from build123d import *

# Parameters (mm, degrees)
SKETCH1_W                  = 38.1
SKETCH1_H                  = 38.1
PRONG_HOLDERS_DEPTH        = 19.05
SKETCH5_R                  = 2.54
SCREW_HOLDER_DEPTH         = 58.15
GROOVE_CUT_OUT_DEPTH       = 58.15
SKETCH6_W                  = 38.1
SKETCH6_H                  = 31.75
OPENING_OF_THE_TOP_DEPTH   = 66.991135768
ROUNDING_OFF_HODER_EDGES_R = 19.05
SKETCH7_W                  = 38.1
SKETCH7_H                  = 38.1
ADJUSTABLE_LENGTH_DEPTH    = 25.4
SKETCH8_W                  = 5.08
SKETCH8_H                  = 38.1
BOSS_EXTRUDE3_DEPTH        = 25.4
SKETCH9_R                  = 2.54
CUT_EXTRUDE4_DEPTH         = 99.578509321


with BuildPart() as part:
    # Sketch1 → Prong holders (new, symmetric)
    with BuildSketch(Plane(origin=(0, 0, 0), x_dir=(1, 0, 0), z_dir=(0, 1, 0))):
        with Locations((19.05, 19.05)):
            Rectangle(SKETCH1_W, SKETCH1_H)
    prong_holders = extrude(amount=PRONG_HOLDERS_DEPTH, both=True)

    # Sketch5 → Screw holder (cut, through all)
    with BuildSketch(Plane(origin=(38.1, 0, 0), x_dir=(0, 0, -1), z_dir=(1, 0, 0))):
        Circle(SKETCH5_R)
    screw_holder = extrude(amount=-SCREW_HOLDER_DEPTH, mode=Mode.SUBTRACT)

    # Sketch4 → Groove cut out (cut, symmetric)
    with BuildSketch(Plane(origin=(0, 0, 0), x_dir=(1, 0, 0), z_dir=(0, 1, 0))):
        Polygon((31.75, 24.13), (29.718, 27.94), (8.382, 27.94), (6.35, 24.13), (6.35, 0), (31.75, 0), align=None)
    groove_cut_out = extrude(amount=GROOVE_CUT_OUT_DEPTH, both=True, mode=Mode.SUBTRACT)

    # Mirror2: Prong holders, Screw holder, Groove cut out across plane
    add(prong_holders.mirror(Plane(origin=(0, 19.05, 0), x_dir=(1, 0, 0), z_dir=(0, 0, -1))))
    add(screw_holder.mirror(Plane(origin=(0, 19.05, 0), x_dir=(1, 0, 0), z_dir=(0, 0, -1))), mode=Mode.SUBTRACT)
    add(groove_cut_out.mirror(Plane(origin=(0, 19.05, 0), x_dir=(1, 0, 0), z_dir=(0, 0, -1))), mode=Mode.SUBTRACT)

    # Sketch6 → Opening of the top (cut, through all)
    with BuildSketch(Plane.XZ.offset(19.05)):
        with Locations((19.05, 22.225)):
            Rectangle(SKETCH6_W, SKETCH6_H)
    extrude(amount=-OPENING_OF_THE_TOP_DEPTH, mode=Mode.SUBTRACT)

    # Rounding off hoder edges
    rounding_off_hoder_edges_edges = [part.edges().sort_by_distance(p)[0] for p in [
        (3.175, 19.05, 6.35),
        (3.175, -19.05, 6.35),
        (34.925, -19.05, 6.35),
        (34.925, 19.05, 6.35),
    ]]
    fillet(rounding_off_hoder_edges_edges, radius=ROUNDING_OFF_HODER_EDGES_R - 0.0001)  # a hair under: the kernel refuses the full size

    # Sketch7 → Adjustable length (add)
    with BuildSketch(Plane(origin=(0, 0, -38.1), x_dir=(-1, 0, 0), z_dir=(0, 0, -1))):
        with Locations((-19.05, 0)):
            Rectangle(SKETCH7_W, SKETCH7_H)
    extrude(amount=ADJUSTABLE_LENGTH_DEPTH)

    # Sketch8 → Boss-Extrude3 (add)
    with BuildSketch(Plane(origin=(0, 0, -63.5), x_dir=(-1, 0, 0), z_dir=(0, 0, -1))):
        with Locations((-35.56, 0)):
            Rectangle(SKETCH8_W, SKETCH8_H)
        with Locations((-2.54, 0)):
            Rectangle(SKETCH8_W, SKETCH8_H)
    extrude(amount=BOSS_EXTRUDE3_DEPTH)

    # Sketch9 → Cut-Extrude4 (cut, through all)
    with BuildSketch(Plane(origin=(38.1, 0, 0), x_dir=(0, 0, -1), z_dir=(1, 0, 0))):
        with Locations((78.74, 0)):
            Circle(SKETCH9_R)
    extrude(amount=-CUT_EXTRUDE4_DEPTH, mode=Mode.SUBTRACT)


solid = part.part
Can you work these out from the model? Positions are in its coordinate system, mm. A direction names the side the tool comes from. Give positions to 0.01 mm unless a question says otherwise; leave off trailing zeros. Order: outer loops, then holes, each group sorted by start corner. A loop starts at its lowest first (then second) coordinate and runs counter-clockwise, first axis right, second up. Notation, with made-up numbers: M -3.75,73 L 15.25,73 A11 cw 15.25,94 Z; hole C -28,83 d11. An arc over 180 degrees is marked long. Use a Markdown table: item, result. Add a question column.
Item 1: Suppose I cut it at C-C (y = 1). Count the separate pieces of the cut face and the enclosed holes in it, then the cut area to 3 significant figures.
Item 2: Suppose I cut it at B-B (z = -23). List the corners of the cut face in (x, y) for me, then the cut area to 3 significant figures.
Item 3: For faces 1 (the cylindrical face through (3.22, 13.32, 0.92)), 2 (the flat face through (31.75, 0, -12)), 3 (the flat face through (33.02, 0, -76)), which set-ups out of +Z, -Z, +X, -X, +Y, -Y let a thin tool reach every point of the face, with its end or its side?
Item 4: Suppose I cut it at A-A (z = -78.74). List the corners of the cut face in (x, y) for me, then the cut area to 3 significant figures.
Item 5: We'd pull the mould along Z, two halves only. Please class faces 4 (the flat face through (5.08, 0, -76)), 5 (the flat face through (36, 0, -88.9)), 6 (the cylindrical face through (35.6, 0.1, -76.2)), 7 (the flat face through (30.748, 0.267, -26.008)): +Z half, -Z half, draft (parallel to the pull), parting line (faces both ways), or undercut.
Item 6: Will these pins go through, and if not, where does the flat tip stop? pin 1 (8 mm diameter, centred on x = 12.5, y = 2.5, fed in from +Z); pin 2 (14 mm diameter, centred on x = 23, y = -7.5, fed in from -Z); pin 3 (12 mm diameter, centred on x = 26.5, y = -10, fed in from +Z).
Item 7: Suppose I cut it at D-D (x = 10). List the corners of the cut face in (y, z) for me.
Item 8: If I drill on L1, parallel to Y at x = 34.55, z = -78.74; L2, parallel to Z at x = 34, y = -1.5; L3, parallel to X at y = -6, z = -22.5, over which ranges is the centre line in solid material (lowest first)? Write a range as [from, to].
Answer sheet:
| question | item | result |
|---|---|---|
| 1 | separate pieces | 5 |
| 1 | enclosed holes | 0 |
| 1 | area | 1,950 mm² |
| 2 | outline | M 0,-19.05 L 6.35,-19.05 L 6.35,19.05 L 0,19.05 Z; M 31.75,-19.05 L 38.1,-19.05 L 38.1,19.05 L 31.75,19.05 Z |
| 2 | area | 484 mm² |
| 3 | face 1 | +Z, +X, -X, +Y |
| 3 | face 2 | +Z, +Y, -Y |
| 3 | face 3 | -Z, +Y, -Y |
| 4 | outline | M 0,-19.05 L 5.08,-19.05 L 5.08,-2.54 L 0,-2.54 Z; M 0,2.54 L 5.08,2.54 L 5.08,19.05 L 0,19.05 Z; M 33.02,-19.05 L 38.1,-19.05 L 38.1,-2.54 L 33.02,-2.54 Z; M 33.02,2.54 L 38.1,2.54 L 38.1,19.05 L 33.02,19.05 Z |
| 4 | area | 335 mm² |
| 5 | face 4 | draft |
| 5 | face 5 | -Z half |
| 5 | face 6 | undercut |
| 5 | face 7 | +Z half |
| 6 | pin 1 | stops at z = -27.94 |
| 6 | pin 2 | stops at z = -63.5 |
| 6 | pin 3 | stops at z = 4.98 |
| 7 | outline | M -19.05,-63.5 L 19.05,-63.5 L 19.05,-27.94 L -19.05,-27.94 Z |
| 8 | L1 | y = [-19.05, -2.54], [2.54, 19.05] |
| 8 | L2 | z = [-88.9, -80.79], [-76.69, -2.05], [2.05, 6.29] |
| 8 | L3 | x = [0, 6.35], [31.75, 38.1] |
